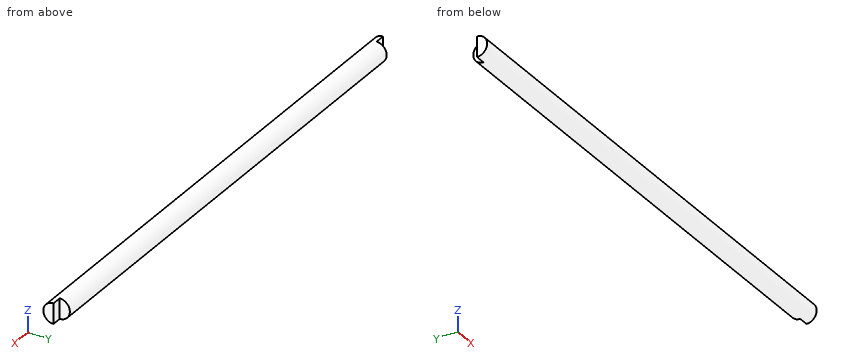
from build123d import *

# Parameters (mm, degrees)
SKETCH1_R               = 6.35
BOSS_EXTRUDE1_DEPTH     = 330.2
SKETCH2_W               = 6.35
SKETCH2_H               = 6.35
CUT_EXTRUDE1_DEPTH      = 7.35
CUT_EXTRUDE1_DEPTH_BACK = 7.35


with BuildPart() as part:
    # Sketch1 → Boss-Extrude1 (new body)
    with BuildSketch(Plane(origin=(0, 0, 0), x_dir=(0, 0, -1), z_dir=(1, 0, 0))):
        Circle(SKETCH1_R)
    extrude(amount=BOSS_EXTRUDE1_DEPTH)

    # Sketch2 → Cut-Extrude1 (cut, two sides)
    with BuildSketch(Plane.XY) as cut_extrude1_sk:
        with Locations((3.175, 3.175)):
            Rectangle(SKETCH2_W, SKETCH2_H)
        with Locations((327.025, 3.175)):
            Rectangle(SKETCH2_W, SKETCH2_H)
    extrude(amount=CUT_EXTRUDE1_DEPTH, mode=Mode.SUBTRACT)
    extrude(cut_extrude1_sk.sketch, amount=-CUT_EXTRUDE1_DEPTH_BACK, mode=Mode.SUBTRACT)


solid = part.part
Check sheet for the modelled part. Datum: model origin and axes. Units: mm. Round coordinates to 2 decimals unless told otherwise and drop trailing zeros. Loops run counter-clockwise (first coordinate to the right, second up) from the corner with the lowest first, then second, coordinate; pieces in that order, holes last. Notation, with made-up numbers: M 62.25,23 L 92.25,23 A32 cw 92.25,62 Z; hole C 75.5,-11 d10. An arc over 180 degrees is marked long. One line per question, with ' | ' between items. Start each with the question number.
Item 1: Section check C-C (x = 242.5). Record the boundary of the cut face in (y, z).
Item 2: Scan lines: probe 1 along X at (y, z) = (0.75, 1.75); probe 2 along Y at (x, z) = (236.5, -0.5); probe 3 along Z at (x, y) = (30, -0.25). Record each from-to range of solid material in increasing order.
Item 3: Section check B-B (y = -4.25). Record the boundary of the cut face in (x, z), and give its area (3 significant figures).
Item 4: Section check A-A (z = 0). Record the boundary of the cut face in (x, y), and give its area (3 significant figures).
Item 5: Gauge pin test, flat ends, axial feed: pin 1 Ø1 at (x, z) = (249, -1) entering from -Y; pin 2 Ø1.9 at (x, z) = (4.5, 0.5) entering from +Y; pin 3 Ø1.9 at (y, z) = (3, -1.5) entering from -X. Record the tip position at first contact, or that the pin passes through.
Worked out:
1) outline: C 0,0 d12.7
2) probe 1: 6.35 to 323.85 | probe 2: -6.33 to 6.33 | probe 3: -6.35 to 6.35
3) outline: M 0,-4.72 L 330.2,-4.72 L 330.2,4.72 L 0,4.72 Z | area: 3,120 mm^2
4) outline: M 0,-6.35 L 330.2,-6.35 L 330.2,0 L 323.85,0 L 323.85,6.35 L 6.35,6.35 L 6.35,0 L 0,0 Z | area: 4,110 mm^2
5) pin 1: y = -6.33 | pin 2: y = 0 | pin 3: x = 6.35
